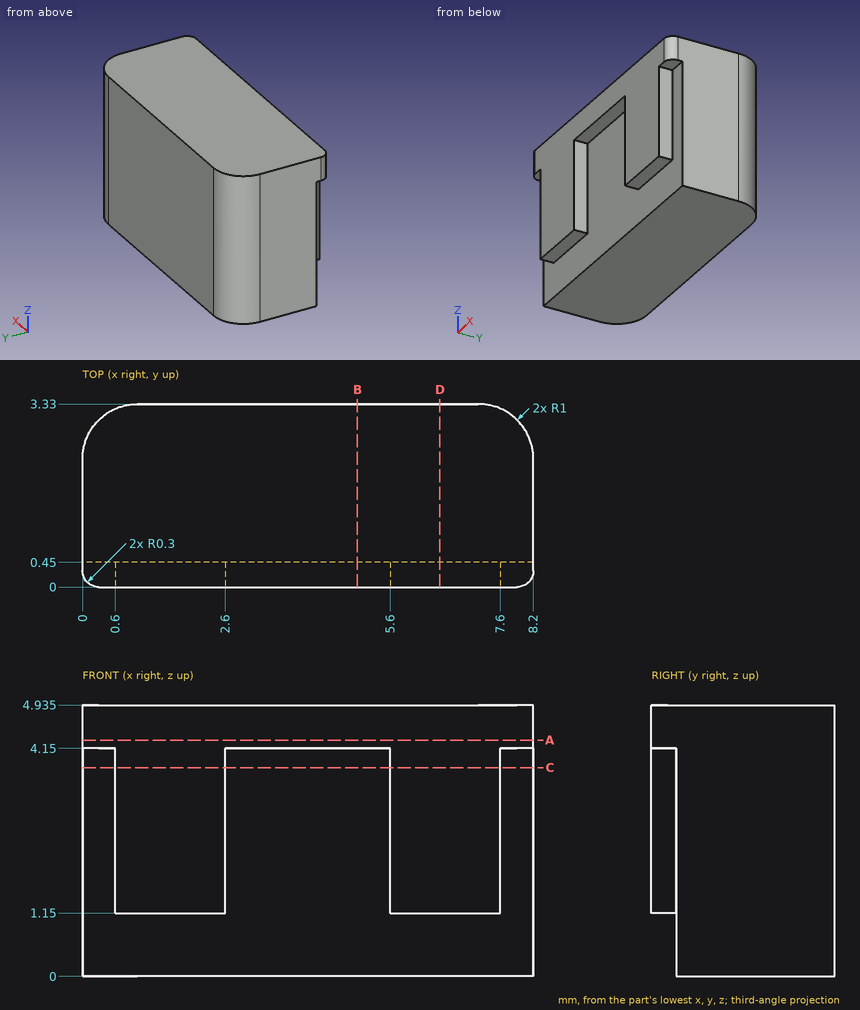
Study the drawing (mm; zero at the part's minimum x, y, z) and answer. Coordinates: 2 decimals unless noted, no trailing zeros. Write each loop counter-clockwise with the first axis right and the second up, starting at its lowest first coordinate (ties: lowest second). Pieces come first, ordered by that corner, then holes. Notation, with made-up numbers: (-35.75, 23) - (-22.75, 23) arc R27 ccw to (-22.75, 62) - close; hole circle Ø8 at (63, -19.75). An arc over 180 degrees is marked (long way). Answer as a JSON object with one key per item and string values. Group by question number.
1. Consider L1, parallel to X at y = 0.4, z = 2.8; L2, parallel to Y at x = 1.25, z = 0.95; L3, parallel to Y at x = 7.5, z = 1.6. Determine where each line is inside the solid, lowest interval first. Write a range as [from, to].
2. A cutting plane is placed at C-C (z = 3.8). Determine the outline of the cut face in (x, y), plus the area to 3 significant figures.
3. A cutting plane is placed at D-D (x = 6.5). Determine the outline of the cut face in (y, z) (3 decimals), plus the area to 3 significant figures.
4. A cutting plane is placed at A-A (z = 4.3). Determine the outline of the cut face in (x, y), plus the area to 3 significant figures.
5. Each of these flat-tipped pins is pushed along its axis until it touches: P1, Ø0.5, axis at y = 0, z = 2, coming from the +X side; P2, Ø1, axis at x = 1.5, z = 0.5, coming from the -Y side. Where does it stop, or does it pass through?
6. A cutting plane is placed at B-B (x = 5). Determine the outline of the cut face in (y, z) (3 decimals).
Worked out:
{
 "1": {"L1": "x = [0.6, 2.6], [5.6, 7.6]", "L2": "y = [0.45, 3.33]", "L3": "y = [0, 3.28]"},
 "2": {"outline": "(0, 0.45) - (0.6, 0.45) - (0.6, 0) - (2.6, 0) - (2.6, 0.45) - (5.6, 0.45) - (5.6, 0) - (7.6, 0) - (7.6, 0.45) - (8.2, 0.45) - (8.2, 2.33) arc R1 ccw to (7.2, 3.33) - (1, 3.33) arc R1 ccw to (0, 2.33) - close", "area": "25.0 mm²"},
 "3": {"outline": "(0, 1.15) - (0.45, 1.15) - (0.45, 0) - (3.33, 0) - (3.33, 4.935) - (0, 4.935) - close", "area": "15.9 mm²"},
 "4": {"outline": "(0, 0.3) arc R0.3 ccw to (0.3, 0) - (7.9, 0) arc R0.3 ccw to (8.2, 0.3) - (8.2, 2.33) arc R1 ccw to (7.2, 3.33) - (1, 3.33) arc R1 ccw to (0, 2.33) - close", "area": "26.8 mm²"},
 "5": {"P1": "stops at x = 7.6", "P2": "stops at y = 0.45"},
 "6": {"outline": "(0, 4.15) - (0.45, 4.15) - (0.45, 0) - (3.33, 0) - (3.33, 4.935) - (0, 4.935) - close"}
}
